Autodesk Inventor part; units mm, degrees
ref_plane "YZ Plane" through (0, 0, 0) normal (1, 0, 0) x (0, 1, 0)
ref_plane "XZ Plane" through (0, 0, 0) normal (0, 1, 0) x (-1, 0, 0)
ref_plane "XY Plane" through (0, 0, 0) normal (0, 0, 1) x (1, 0, 0)
sketch "Sketch1" plane through (0, 0, 0) normal (0, 0, 1) x (1, 0, 0)
  line L0 (0, 0) -> (101.6, 0)
  line L1 (101.6, 0) -> (101.6, 63.5)
  line L2 (101.6, 63.5) -> (0, 63.5)
  line L3 (0, 63.5) -> (0, 0)
  dimension "d0" = 101.6
  dimension "d1" = 63.5
extrude "Extrusion1" add sketch "Sketch1" along normal blind 25.4
sketch "Sketch2" plane through (101.6, 0, 0) normal (1, 0, 0) x (0, 0, -1)
  circle A0 centre (-12.7, 44.45) radius 6.35
  line L0 (-25.4, 0) -> (-25.4, 63.5)
  line L1 (0, 0) -> (-25.4, 0)
  line L2 (0, 63.5) -> (-25.4, 63.5)
  dimension "d4" = 12.7
  dimension "d5" = 12.7
  dimension "d13" = 19.05
extrude "Extrusion2" cut sketch "Sketch2" against normal blind 101.6
sketch "Sketch3" plane through (0, 63.5, 0) normal (0, 1, 0) x (1, 0, 0)
  line L0 (0, -25.4) -> (101.6, -25.4)
  line L1 (0, 0) -> (101.6, 0)
  line L2 (39.37, -25.4) -> (62.23, -25.4)
  line L3 (62.23, -25.4) -> (62.23, 0)
  line L4 (62.23, 0) -> (39.37, 0)
  line L5 (39.37, 0) -> (39.37, -25.4)
  line L6 (101.6, 0) -> (101.6, -25.4)
  dimension "d9" = 22.86
  dimension "d10" = 39.37
extrude "Extrusion3" cut sketch "Sketch3" against normal blind 60.96 contours L5 L1 L3 L0
properties part number "Kermit MountConnectors"
The model under review builds one solid part; all positions refer to its coordinate system, in mm. A direction names the side the tool comes from. Round coordinates to 2 decimals unless told otherwise and drop trailing zeros. Order: outer loops, then holes, each group sorted by start corner. A loop starts at its lowest first (then second) coordinate and runs counter-clockwise, first axis right, second up.
(1) Take a section at B-B, the plane z = 12.7. State the section outline as (x, y) points.
Working result:
outline: (0, 0) - (101.6, 0) - (101.6, 38.1) - (62.23, 38.1) - (62.23, 2.54) - (39.37, 2.54) - (39.37, 38.1) - (0, 38.1) - close; (0, 50.8) - (39.37, 50.8) - (39.37, 63.5) - (0, 63.5) - close; (62.23, 50.8) - (101.6, 50.8) - (101.6, 63.5) - (62.23, 63.5) - close
(2) Take a section at D-D, the plane x = 8. State the section outline as (y, z) points, plus the area to 3 significant figures.
Working result:
outline: (0, 0) - (63.5, 0) - (63.5, 25.4) - (0, 25.4) - close; hole circle Ø12.7 at (44.45, 12.7)
area: 1,490 mm2
(3) Take a section at C-C, the plane y = 44.45. State the section outline as (x, z) points.
Working result:
outline: (0, 0) - (39.37, 0) - (39.37, 6.35) - (0, 6.35) - close; (0, 19.05) - (39.37, 19.05) - (39.37, 25.4) - (0, 25.4) - close; (62.23, 0) - (101.6, 0) - (101.6, 6.35) - (62.23, 6.35) - close; (62.23, 19.05) - (101.6, 19.05) - (101.6, 25.4) - (62.23, 25.4) - close
(4) Mouldability with a two-part tool opening along X and no side actions: class faces 3 (the face through (19.961, 50.746, 13.527)), 4 (the face through (0, 32, 13)), 5 (the face through (62.23, 33, 13)) as released by +X, released by -X, zero draft, split by the parting line, or undercut.
Working result:
face 3: zero draft
face 4: released by -X
face 5: undercut
(5) Tool access review of faces 1 (the face through (51, 2.54, 13)), 2 (the face through (39, 32, 25.4)): name each direction out of +Z, -Z, +X, -X, +Y, -Y from which nothing blocks a thin tool from reaching the whole face with its end or side.
Working result:
face 1: +Z, -Z, +Y
face 2: +Z, +X, -X, +Y, -Y
(6) For P1, Ø8, axis at x = 53.5, z = 7.5, coming from the +Y side, flat-tipped, find the tip position at first contact; note if it passes through.
Working result:
P1: stops at y = 2.54
(7) Wall thickness on L1, parallel to X at y = 22.5, z = 10; L2, parallel to Y at x = 77.5, z = 12.7; L3, parallel to Z at x = 13, y = 44: over which ranges is each line inside the solid? List them lowest first.
Working result:
L1: x = 0 to 39.37, 62.23 to 101.6
L2: y = 0 to 38.1, 50.8 to 63.5
L3: z = 0 to 6.37, 19.03 to 25.4
(8) Take a section at A-A, the plane y = 12. State the section outline as (x, z) points, plus the area to 3 significant figures.
Working result:
outline: (0, 0) - (39.37, 0) - (39.37, 25.4) - (0, 25.4) - close; (62.23, 0) - (101.6, 0) - (101.6, 25.4) - (62.23, 25.4) - close
area: 2,000 mm2
